from build123d import *

# Parameters (mm, degrees)
F0_R         = 42.8944136966
F1_DEPTH     = 7.62
F2_W         = 53.9315019637
F2_H         = 50.8
F3_DEPTH     = 25.4
F4_DEPTH     = 127
F5_R         = 42.3296228718
F6_DEPTH     = 7.62
F7_R         = 23.1378072787
F8_DEPTH     = 5.08
F9_R         = 24.1805765137
F10_DEPTH    = 5.08
F11_T1_DEPTH = 25.4


# Not quite as in the source:
# - a fillet or chamfer that OpenCascade refuses, or shapes differently, is made with other operations: its cross-section is extruded or revolved along the edge and cut away or added


with BuildPart() as f1:
    # F0 (on Right) → F1 (new body)
    with BuildSketch(Plane.YZ):
        Circle(F0_R)
    extrude(amount=F1_DEPTH)

    # F2 (on face) → F3 (join)
    with BuildSketch(Plane(origin=(0, 0, 0), x_dir=(0, -1, 0), z_dir=(-1, 0, 0))):
        with Locations((0.0807167962, 0.2214573324)):
            Rectangle(F2_W, F2_H)
    extrude(amount=F3_DEPTH)

    # F4 (add): a face of the model
    f4_faces = [f1.faces().sort_by_distance(p)[0] for p in [
        (-12.7, -27.0464677781, 0.2214573324),
    ]]
    extrude(f4_faces, amount=F4_DEPTH)

    # F5 (on face) → F6 (join)
    with BuildSketch(Plane(origin=(-25.4, 0, 0), x_dir=(0, -1, 0), z_dir=(-1, 0, 0))):
        with Locations((2.3584635928, 0)):
            Circle(F5_R)
    extrude(amount=F6_DEPTH)

    # F7 (on face) → F8 (join)
    with BuildSketch(Plane(origin=(-25.4, 0, 0), x_dir=(0, -1, 0), z_dir=(-1, 0, 0))):
        with Locations((154.0464677781, -14.1031453386)):
            Circle(F7_R)
    extrude(amount=F8_DEPTH)

    # F9 (on face) → F10 (join)
    with BuildSketch(Plane.YZ):
        with Locations((-154.0464677781, -11.9213024154)):
            Circle(F9_R)
    extrude(amount=F10_DEPTH)

    # F11: chamfer of 152.4 x 26.87223186 on 1 edges, made by hand

    # F11_s2 → F11_t1 (cut)
    with BuildSketch(Plane.YZ.offset(-25.4)):
        Polygon((-1.6464677781, 25.6214573324), (-154.0464677781, -1.2507745276), (-154.0464677781, 25.6214573324), align=None)
    extrude(amount=F11_T1_DEPTH, mode=Mode.SUBTRACT)


solid = f1.part
Read the model definition and answer for the solid it produces. Units are mm, in the model's axes. A direction names the side the tool comes from. Round coordinates to 2 decimals unless told otherwise and drop trailing zeros. Order: outer loops, then holes, each group sorted by start corner. A loop starts at its lowest first (then second) coordinate and runs counter-clockwise, first axis right, second up.
1) Straight lines are drawn through the part: L1, parallel to X at y = -21, z = -27; L2, parallel to Z at x = -22, y = -154; L3, parallel to X at y = -65.5, z = 8. For each, find the intervals that lie inside material, in ascending order.
2) The part is cut by section C-C on x = -4. Write down the section's boundary in (y, z), plus the area to 3 significant figures.
3) Flat-ended cylindrical pins translate along their axes: pin 1 (20.5 mm diameter, centred on x = -7.5, y = -101.5, fed in from -Z); pin 2 (13 mm diameter, centred on y = -151.5, z = -6, fed in from +X); pin 3 (12 mm diameter, centred on x = -9, y = -98.5, fed in from +Z). Find the tip coordinate at first contact, or state that the pin passes through.
4) For faces 1 (the face through (-13, -62, -25.179)), 2 (the face through (-30.48, -154, -14)), 3 (the face through (-13, 13, 25.621)), 4 (the face through (-13, -154.046, -13)), 5 (the face through (-27.9, -130.93, -13.09)), determine the directions among +Z, -Z, +X, -X, +Y, -Y from which every point of the face is accessible in a straight line to the end or side of a thin tool.
5) The part is cut by section D-D on y = 0.5. Write down the section's boundary in (x, z).
6) The part is cut by section A-A on y = -165. Write down the section's boundary in (x, z), plus the area to 3 significant figures.
7) The part is cut by section B-B on z = 38.5. Write down the section's boundary in (x, y).
8) The mould has two halves that part along Y. Classify faces 6 (the face through (2.504, -178.204, -10.858)), 7 (the face through (5.08, -154, -12)), 8 (the face through (-13, 26.885, 0)): released by +Y, released by -Y, zero draft, split by the parting line, or undercut.
Resolved:
1. L1: x = -33.02 to -25.4, 0 to 7.62
1. L2: z = -25.18 to -1.24
1. L3: x = -25.4 to 0
2. outline: (-154.05, -25.18) - (26.89, -25.18) - (26.89, 25.62) - (-1.65, 25.62) - (-154.05, -1.25) - close
2. area: 7,140 mm2
3. pin 1: stops at z = -25.18
3. pin 2: stops at x = 5.08
3. pin 3: stops at z = 9.6
4. face 1: -Z, +Y, -Y
4. face 2: +Z, -Z, -X, -Y
4. face 3: +Z, +Y, -Y
4. face 4: +Z, -Z, -Y
4. face 5: -X
5. outline: (-33.02, -42.23) - (-25.4, -42.23) - (-25.4, -25.18) - (0, -25.18) - (0, -42.89) - (7.62, -42.89) - (7.62, 42.89) - (0, 42.89) - (0, 25.62) - (-25.4, 25.62) - (-25.4, 42.23) - (-33.02, 42.23) - close
6. outline: (-30.48, -34.48) - (-25.4, -34.48) - (-25.4, 6.28) - (-30.48, 6.28) - close; (0, -33.48) - (5.08, -33.48) - (5.08, 9.64) - (0, 9.64) - close
6. area: 426 mm2
7. outline: (-33.02, -19.95) - (-25.4, -19.95) - (-25.4, 15.24) - (-33.02, 15.24) - close; (0, -18.91) - (7.62, -18.91) - (7.62, 18.91) - (0, 18.91) - close
8. face 6: undercut
8. face 7: zero draft
8. face 8: released by +Y
